```python
from build123d import *

# Parameters (mm, degrees)
EXTRUDE_1_DEPTH = 1
SKETCH_2_W      = 3.1
SKETCH_2_H      = 3.3
EXTRUDE_2_DEPTH = 0.83
SKETCH_3_W      = 4.4
SKETCH_3_H      = 1
SKETCH_3_W_2    = 0.8
SKETCH_3_H_2    = 1.5
EXTRUDE_3_DEPTH = 1
FILLET_1_R      = 1


with BuildPart() as part:
    # 草图1 → 凸台-拉伸1 (new body)
    with BuildSketch(Plane(origin=(0, 0, 0), x_dir=(1, 0, 0), z_dir=(0, 1, 0))):
        with BuildLine():
            Line((0, 0), (9.05, 0))
            Line((9.05, 0), (9.05, -0.85))
            ThreePointArc((9.05, -0.85), (9.8, -1.6), (10.55, -0.85))
            Line((10.55, -0.85), (10.55, 0))
            Line((10.55, 0), (19.6, 0))
            Line((19.6, 0), (19.6, -9))
            Line((19.6, -9), (10.55, -9))
            Line((10.55, -9), (10.55, -8.15))
            ThreePointArc((10.55, -8.15), (9.8, -7.4), (9.05, -8.15))
            Line((9.05, -8.15), (9.05, -9))
            Line((9.05, -9), (0, -9))
            Line((0, -9), (0, 0))
        make_face()
    extrude(amount=EXTRUDE_1_DEPTH)

    # 草图2 → 凸台-拉伸2 (add)
    with BuildSketch(Plane(origin=(0, 1, 0), x_dir=(1, 0, 0), z_dir=(0, 1, 0))):
        with Locations((3.85, -4.5)):
            Rectangle(SKETCH_2_W, SKETCH_2_H)
        with Locations((7.5, -4.5)):
            Rectangle(SKETCH_2_W, SKETCH_2_H)
        with Locations((12.1, -4.5)):
            Rectangle(SKETCH_2_W, SKETCH_2_H)
        with Locations((15.75, -4.5)):
            Rectangle(SKETCH_2_W, SKETCH_2_H)
    extrude(amount=EXTRUDE_2_DEPTH)

    # 草图3 → 凸台-拉伸3 (add)
    with BuildSketch(Plane(origin=(0, 1, 0), x_dir=(1, 0, 0), z_dir=(0, 1, 0))):
        with Locations((17.4, -7.3)):
            Rectangle(SKETCH_3_W, SKETCH_3_H)
        with Locations((9.8, -4.5)):
            Rectangle(SKETCH_3_W_2, SKETCH_3_H_2)
        with Locations((17.4, -1.7)):
            Rectangle(SKETCH_3_W, SKETCH_3_H)
    extrude(amount=EXTRUDE_3_DEPTH)

    # 圆角1
    fillet_1_edges = [part.edges().sort_by_distance(p)[0] for p in [
        (19.6, 2, 7.3),
        (19.6, 2, 1.7),
    ]]
    fillet(fillet_1_edges, radius=FILLET_1_R)


solid = part.part
```
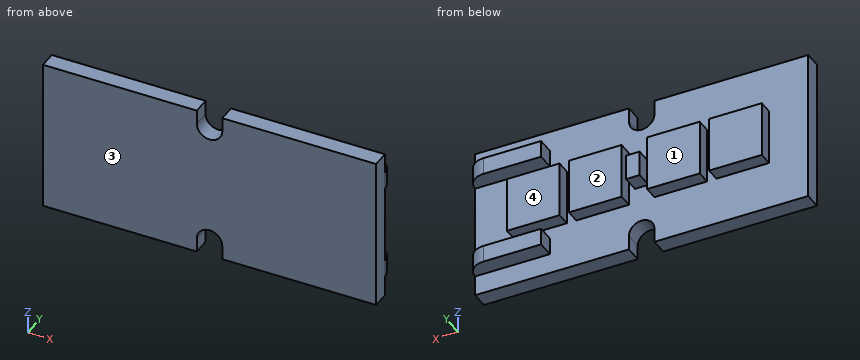
Work out the finished part from the listing and answer in its coordinate system (mm). Face numbers are marked on the shaded views. A direction names the side the tool comes from. Round coordinates to 2 decimals unless told otherwise and drop trailing zeros. Loops run counter-clockwise (first coordinate to the right, second up) from the corner with the lowest first, then second, coordinate; pieces in that order, holes last.
(1) The part is cut by section D-D, the plane y = 0.45. Give the vertices of the cut face in (x, z).
Computed values:
outline: (0, 0) - (9.05, 0) - (9.05, 0.85) arc R0.75 cw to (10.55, 0.85) - (10.55, 0) - (19.6, 0) - (19.6, 9) - (10.55, 9) - (10.55, 8.15) arc R0.75 cw to (9.05, 8.15) - (9.05, 9) - (0, 9) - close
(2) The part is cut by section A-A, the plane z = 8.5. Give the vertices of the cut face in (x, y).
Computed values:
outline: (0, 0) - (9.05, 0) - (9.05, 1) - (0, 1) - close; (10.55, 0) - (19.6, 0) - (19.6, 1) - (10.55, 1) - close
(3) The mould has two halves that part along Z. Classify the marked faces 3 and 4: pulls with the +Z half, pulls with the -Z half, needs draft (parallel to the pull), parting line crosses it, or undercut.
Computed values:
face 3: needs draft
face 4: undercut
(4) Find the intervals of material crossed by L1, parallel to X at y = 1.45, z = 3.25; L2, parallel to X at y = 1.6, z = 4.5; L3, parallel to Z at x = 18, y = 1.95, in increasing order.
Computed values:
L1: x = 2.3 to 5.4, 5.95 to 9.05, 10.55 to 13.65, 14.2 to 17.3
L2: x = 2.3 to 5.4, 5.95 to 9.05, 9.4 to 10.2, 10.55 to 13.65, 14.2 to 17.3
L3: z = 1.2 to 2.2, 6.8 to 7.8
(5) The part is cut by section B-B, the plane x = 14.5. Give the vertices of the cut face in (y, z).
Computed values:
outline: (0, 0) - (1, 0) - (1, 2.85) - (1.83, 2.85) - (1.83, 6.15) - (1, 6.15) - (1, 9) - (0, 9) - close
(6) The part is cut by section C-C, the plane y = 1.55. Give the vertices of the cut face in (x, z).
Computed values:
outline: (2.3, 2.85) - (5.4, 2.85) - (5.4, 6.15) - (2.3, 6.15) - close; (5.95, 2.85) - (9.05, 2.85) - (9.05, 6.15) - (5.95, 6.15) - close; (9.4, 3.75) - (10.2, 3.75) - (10.2, 5.25) - (9.4, 5.25) - close; (10.55, 2.85) - (13.65, 2.85) - (13.65, 6.15) - (10.55, 6.15) - close; (14.2, 2.85) - (17.3, 2.85) - (17.3, 6.15) - (14.2, 6.15) - close; (15.2, 1.2) - (19.44, 1.2) - (19.44, 2.2) - (15.2, 2.2) - close; (15.2, 6.8) - (19.44, 6.8) - (19.44, 7.8) - (15.2, 7.8) - close
(7) Each of these flat-tipped pins is pushed along its axis until it touches: P1, Ø0.5, axis at x = 16.5, y = 1.5, coming from the +Z side; P2, Ø0.5, axis at y = 1.5, z = 7.5, coming from the -X side; P3, Ø0.6, axis at x = 10, y = 1.5, coming from the -Z side. Where does it stop, or does it pass through?
Computed values:
P1: stops at z = 7.8
P2: stops at x = 15.2
P3: stops at z = 3.75
(8) For the marked faces 1 and 2, determine the directions among +Z, -Z, +X, -X, +Y, -Y from which every point of the face is accessible in a straight line to the end or side of a thin tool.
Computed values:
face 1: +Z, -Z, -X, +Y
face 2: +Z, -Z, +X, +Y
